Geometry check sheet. Reference: the model listing, model coordinates, mm. A direction names the side the tool comes from. Coordinates: 2 decimals unless noted, no trailing zeros. Write each loop counter-clockwise with the first axis right and the second up, starting at its lowest first coordinate (ties: lowest second). Pieces come first, ordered by that corner, then holes. Notation, with made-up numbers: M 32.5,-6.75 L 62.5,-6.75 A18 cw 62.5,17.25 Z; hole C 38,67 d9. An arc over 180 degrees is marked long. Put each result on its own line as item: value. Start each with the question number.
1) Cross-section at D-D on x = -34.5. Record the cut outline in (y, z).
2) Cross-section at A-A on y = 23.5. Record the cut outline in (x, z).
3) Scan lines: line 1 along Y through (x, z) = (-65, -21.75); line 2 along Z through (x, y) = (52, 14); line 3 along X through (y, z) = (10.5, -27). Record each from-to range of solid material in increasing order.
4) Cross-section at C-C on x = -66. Record the cut outline in (y, z).
5) Gauge pin test, flat ends, axial feed: pin 1 (13 mm diameter, centred on x = -61.5, y = 13, fed in from -Z); pin 2 (19.5 mm diameter, centred on x = 34.5, z = 13, fed in from +Y); pin 3 (2.5 mm diameter, centred on y = 8, z = -23, fed in from +X). Record the tip position at first contact, or that the pin passes through.
6) Mould release check, pull along X, two halves, no side actions. Record for faces 4 (the flat face through (17, 15, -35)), 5 (the flat face through (75, 0, 1)), 6 (the flat face through (-72.973, 6, 0)): released by +X, released by -X, zero draft, split by the parting line, or undercut.
7) Cross-section at B-B on z = 0. Record the cut outline in (x, y), plus the area to 3 significant figures.
8) Set-up check for faces 1 (the flat face through (69.663, 18.191, -0.455)), 2 (the cylindrical face through (13.368, 13.592, 6.349)), 3 (the flat face through (0, 25, 0)): record each of +Z, -Z, +X, -X, +Y, -Y from which the full face is reachable in a straight line by a thin tool's end or side.
from build123d import *

# Parameters (mm, degrees)
SKETCH1_W               = 150
SKETCH1_H               = 75
BOSS_EXTRUDE1_DEPTH     = 2.5
BOSS_EXTRUDE5_START     = 32.5
BOSS_EXTRUDE5_DEPTH     = 2.5
BOSS_EXTRUDE2_START     = 17.5
SKETCH3_R               = 4
BOSS_EXTRUDE2_DEPTH     = 15
SKETCH2_R               = 10
SKETCH2_R_2             = 8
BOSS_EXTRUDE3_DEPTH     = 22.5
SKETCH5_W               = 2.026540741
SKETCH5_H               = 65
BOSS_EXTRUDE4_DEPTH     = 7.25
BOSS_EXTRUDE6_DEPTH     = 65
CUT_EXTRUDE1_DEPTH      = 112.106096906
CUT_EXTRUDE1_DEPTH_BACK = 112.106096906
SKETCH9_R               = 4
SKETCH13_R              = 2.5
CUT_EXTRUDE4_DEPTH      = 5


with BuildPart() as part:
    # Sketch1 → Boss-Extrude1 (new, symmetric)
    with BuildSketch(Plane(origin=(0, 0, 0), x_dir=(1, 0, 0), z_dir=(0, 1, 0))):
        Rectangle(SKETCH1_W, SKETCH1_H)
    extrude(amount=BOSS_EXTRUDE1_DEPTH, both=True)

    # Sketch7 → Boss-Extrude5 (add)
    with BuildSketch(Plane.XY.offset(BOSS_EXTRUDE5_START)):
        Polygon((70.01742626, 34.649589392), (74.25, 2.5), (-75, 2.5), (-76.731484571, 15.635393826), align=None)
    boss_extrude5 = extrude(amount=BOSS_EXTRUDE5_DEPTH)

    # Sketch3 → Boss-Extrude2 (add)
    with BuildSketch(Plane.XY.offset(BOSS_EXTRUDE2_START)):
        with BuildLine():
            Line((-72.973459259, 2.5), (-72.973459259, 11.15111247))
            ThreePointArc((-72.973459259, 11.15111247), (-65, 18.5), (-57.026540741, 11.15111247))
            Line((-57.026540741, 11.15111247), (-57.026540741, 2.5))
            Line((-57.026540741, 2.5), (-72.973459259, 2.5))
        make_face()
        with Locations(Location((-65, 10.5, 0), (0, 0, 180))):
            Circle(SKETCH3_R, mode=Mode.SUBTRACT)
    boss_extrude2 = extrude(amount=BOSS_EXTRUDE2_DEPTH)

    # Mirror1: Boss-Extrude5, Boss-Extrude2 across plane
    add(boss_extrude5.mirror(Plane.XY))
    add(boss_extrude2.mirror(Plane.XY))

    # Sketch2 → Boss-Extrude3 (add)
    with BuildSketch(Plane(origin=(0, 2.5, 0), x_dir=(1, 0, 0), z_dir=(0, 1, 0))):
        with Locations(Location((8.5, 0, 0), (0, 0, 90))):
            Circle(SKETCH2_R)
        with Locations(Location((8.5, 0, 0), (0, 0, 90))):
            Circle(SKETCH2_R_2, mode=Mode.SUBTRACT)
    extrude(amount=BOSS_EXTRUDE3_DEPTH)

    # Sketch5 → Boss-Extrude4 (add)
    with BuildSketch(Plane(origin=(0, 2.5, 0), x_dir=(1, 0, 0), z_dir=(0, 1, 0))):
        with Locations((-73.98672963, 0)):
            Rectangle(SKETCH5_W, SKETCH5_H)
    extrude(amount=BOSS_EXTRUDE4_DEPTH)

    # Sketch8 → Boss-Extrude6 (add)
    with BuildSketch(Plane.XY.offset(-32.5)):
        Polygon((70.01742626, 34.649589392), (74.25, 2.5), (71.728427599, 2.5), (67.53814582, 34.328350053), align=None)
    extrude(amount=BOSS_EXTRUDE6_DEPTH)

    # Sketch9 → Cut-Extrude1 (cut, two sides: drawn at the far end of the back side and taken through both)
    with BuildSketch(Plane.XY.offset(35).offset(-CUT_EXTRUDE1_DEPTH_BACK)):
        with Locations(Location((-65, 10.5, 0), (0, 0, 180))):
            Circle(SKETCH9_R)
    extrude(amount=CUT_EXTRUDE1_DEPTH + CUT_EXTRUDE1_DEPTH_BACK, mode=Mode.SUBTRACT)

    # Sketch13 → Cut-Extrude4 (cut)
    with BuildSketch(Plane(origin=(73.308520107, 9.651249767, 0), x_dir=(0, 0, -1), z_dir=(0.9914448613738098, 0.13052619222005604, 0))):
        with Locations(Location((0, -2.212957619, 0), (0, 0, 90))):
            Circle(SKETCH13_R)
    extrude(amount=-CUT_EXTRUDE4_DEPTH, mode=Mode.SUBTRACT)


solid = part.part
Answer key:
1. outline: M -2.5,-37.5 L 2.5,-37.5 L 2.5,-35 L 21.11,-35 L 21.11,-32.5 L 2.5,-32.5 L 2.5,32.5 L 21.11,32.5 L 21.11,35 L 2.5,35 L 2.5,37.5 L -2.5,37.5 Z
2. outline: M -16.03,-35 L 71.49,-35 L 71.49,35 L -16.03,35 L -16.03,32.5 L 68.96,32.5 L 68.96,-32.5 L -16.03,-32.5 Z; C 8.5,0 d20; hole C 8.5,0 d16
3. line 1: y = -2.5 to 6.5, 14.5 to 18.5
3. line 2: z = -35 to -32.5, 32.5 to 35
3. line 3: x = -72.97 to -69, -61 to -57.03, 70.68 to 73.2
4. outline: M -2.5,-37.5 L 2.5,-37.5 L 2.5,-35 L 6.63,-35 L 6.63,-17.5 L 2.5,-17.5 L 2.5,17.5 L 6.63,17.5 L 6.63,35 L 2.5,35 L 2.5,37.5 L -2.5,37.5 Z; M 14.37,-35 L 17.03,-35 L 17.03,-32.5 L 18.44,-32.5 L 18.44,-17.5 L 14.37,-17.5 Z; M 14.37,17.5 L 18.44,17.5 L 18.44,32.5 L 17.03,32.5 L 17.03,35 L 14.37,35 Z
5. pin 1: stops at z = -35
5. pin 2: stops at y = 2.5
5. pin 3: stops at x = 73.69
6. face 4: zero draft
6. face 5: released by +X
6. face 6: undercut
7. outline: M -75,-2.5 L 75,-2.5 L 75,2.5 L 74.25,2.5 L 73.92,4.98 L 71.45,4.65 L 71.73,2.5 L 18.5,2.5 L 18.5,25 L 16.5,25 L 16.5,2.5 L 0.5,2.5 L 0.5,25 L -1.5,25 L -1.5,2.5 L -72.97,2.5 L -72.97,9.75 L -75,9.75 Z; M 67.54,34.33 L 70.79,9.61 L 73.27,9.94 L 70.02,34.65 Z
7. area: 923 mm²
8. face 1: none
8. face 2: +Y
8. face 3: -X, +Y
